Source: three-view drawing plus pictorial views. Frame: mm from the lowest corner of the part. Coordinates: 2 decimals unless noted, no trailing zeros. Write each loop counter-clockwise with the first axis right and the second up, starting at its lowest first coordinate (ties: lowest second). Pieces come first, ordered by that corner, then holes. Notation, with made-up numbers: (36, 46) - (92, 46) arc R24 ccw to (92, 62) - close; hole circle Ø8 at (34.25, -9.5). An arc over 180 degrees is marked (long way). One line per item, written item: value.
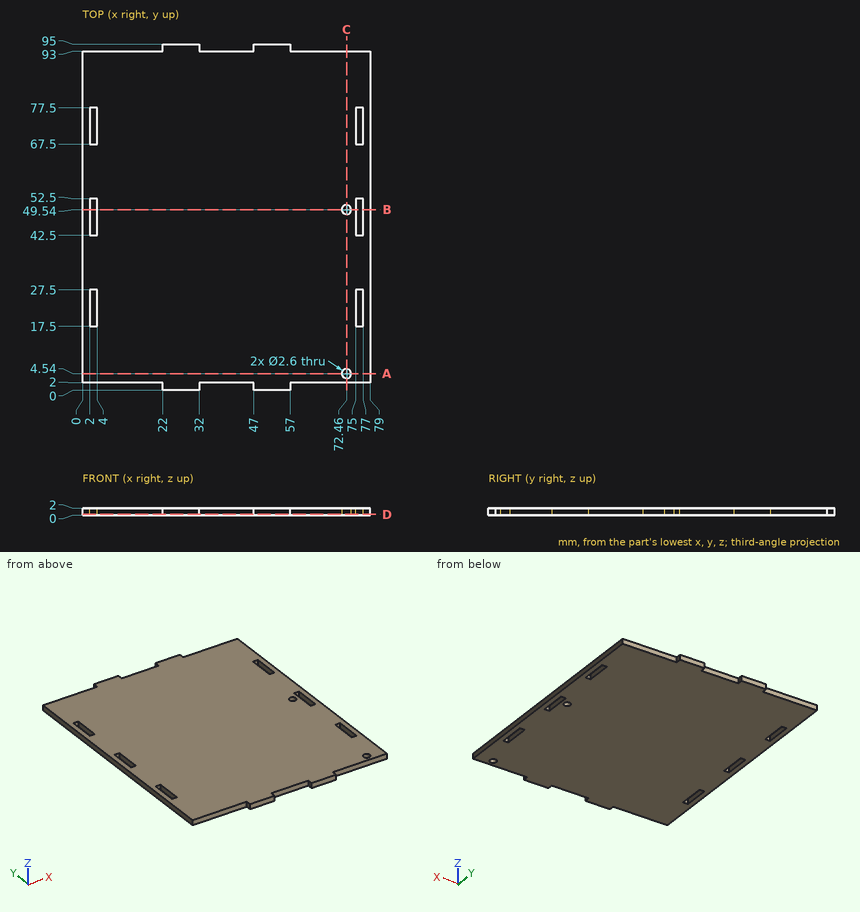
1) Section query C-C on x = 72.46. Output: boundary loops of the cut face in (y, z), then the cut area to 3 significant figures.
Values found:
outline: (2, 0) - (3.24, 0) - (3.24, 2) - (2, 2) - close; (5.84, 0) - (48.24, 0) - (48.24, 2) - (5.84, 2) - close; (50.84, 0) - (93, 0) - (93, 2) - (50.84, 2) - close
area: 172 mm2
2) Section query A-A on y = 4.54. Output: boundary loops of the cut face in (x, z).
Values found:
outline: (0, 0) - (71.16, 0) - (71.16, 2) - (0, 2) - close; (73.76, 0) - (79, 0) - (79, 2) - (73.76, 2) - close
3) Contact query for flat-ended pins moving along their axis: P1, Ø3, axis at x = 72.46, y = 49.54, coming from the +Z side; P2, Ø1, axis at x = 69.5, z = 1, coming from the +Y side; P3, Ø1, axis at x = 76.5, z = 1.5, coming from the -Y side. Output: stop coordinate, or through.
Values found:
P1: z = 2
P2: y = 93
P3: y = 2
4) Material intervals for line 1 (X direction, y = 27, z = 0.25); line 2 (Y direction, x = 72.46, z = 0.7); line 3 (X direction, y = 48.5, z = 1.8), sorted ascending.
Values found:
line 1: 0 to 2, 4 to 75, 77 to 79
line 2: 2 to 3.24, 5.84 to 48.24, 50.84 to 93
line 3: 0 to 2, 4 to 71.68, 73.24 to 75, 77 to 79
5) Section query B-B on y = 49.54. Output: boundary loops of the cut face in (x, z).
Values found:
outline: (0, 0) - (2, 0) - (2, 2) - (0, 2) - close; (4, 0) - (71.16, 0) - (71.16, 2) - (4, 2) - close; (73.76, 0) - (75, 0) - (75, 2) - (73.76, 2) - close; (77, 0) - (79, 0) - (79, 2) - (77, 2) - close
6) Section query D-D on z = 0.3. State how many separate pieces and enclosed holes the cut face has, then the cut area to 3 significant figures.
Values found:
separate pieces: 1
enclosed holes: 8
area: 7,140 mm2
